Part print with two shaded views. Sizes in mm from the minimum x, y, z corner. Round coordinates to 2 decimals unless told otherwise and drop trailing zeros. Loops run counter-clockwise (first coordinate to the right, second up) from the corner with the lowest first, then second, coordinate; pieces in that order, holes last. Notation, with made-up numbers: (-33.5, 79) -> (22.5, 79) arc R24 ccw to (22.5, 100) -> close; hole circle Ø6 at (32, 41). An arc over 180 degrees is marked (long way). Use a Markdown table: item, result. Add a question column.
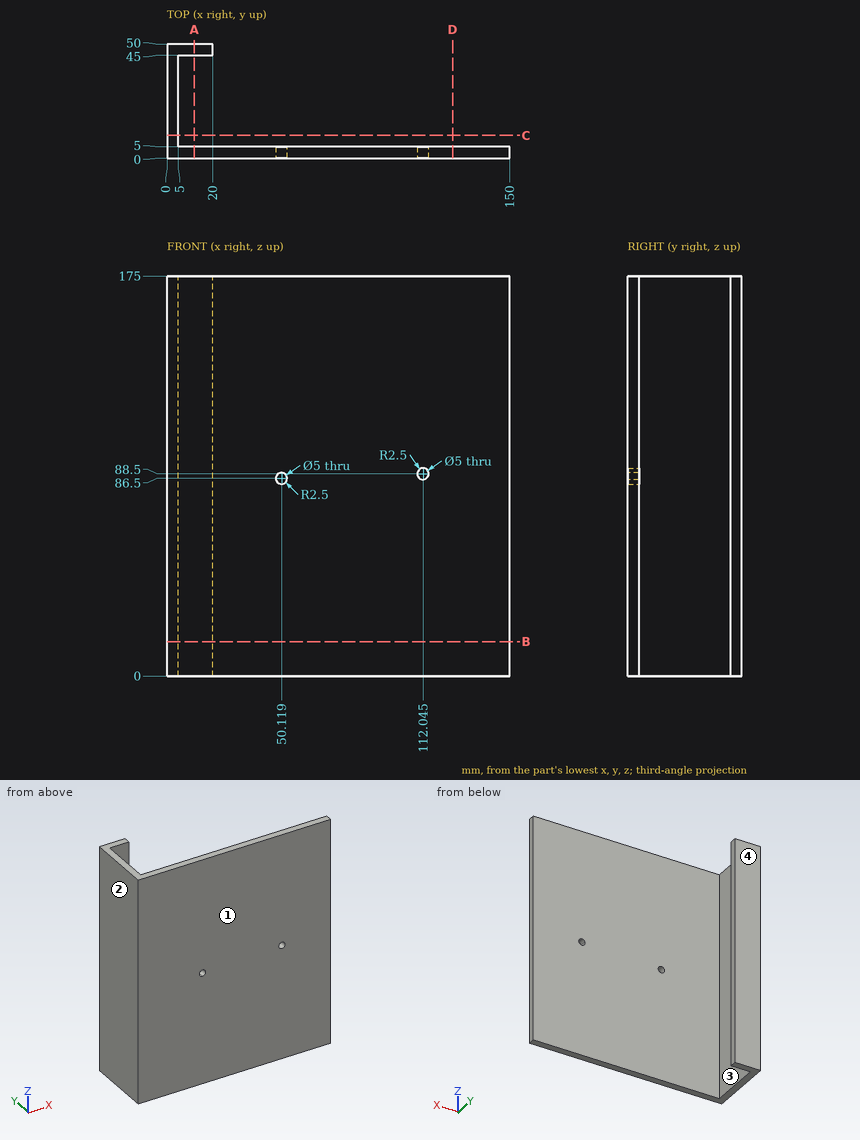
1) Cut at A-A on x = 12. Write the cut outline in (y, z).
2) Pull direction Y, two halves, no side cores. Call the marked faces 1, 2, 3 and 4: +Y half, -Y half, draft (parallel to the pull), parting line (faces both ways), or undercut.
3) Cut at B-B on z = 15. Write the cut outline in (x, y), and give its area (3 significant figures).
4) Cut at C-C on y = 10. Write the cut outline in (x, z), and give its area (3 significant figures).
5) Wall check: probe 1 along X at (y, z) = (2, 88.5) (1 decimal); probe 2 along X at (y, z) = (2, 88) (1 decimal); probe 3 along Y at (x, z) = (130.5, 32). Give the ranges that are in metal, low to high. Write a range as from..to.
6) Pin check, flat tips, straight feed: pin 1 Ø12 at (y, z) = (27.5, 135) entering from -X; pin 2 Ø20 at (y, z) = (19.5, 56) entering from +X; pin 3 Ø4 at (y, z) = (48, 61) entering from +X; pin 4 Ø8 at (x, z) = (57.5, 151.5) entering from +Y. Stop position of each tip, or through.
Established:
| question | item | result |
|---|---|---|
| 1 | outline | (0, 0) -> (5, 0) -> (5, 175) -> (0, 175) -> close; (45, 0) -> (50, 0) -> (50, 175) -> (45, 175) -> close |
| 2 | face 1 | -Y half |
| 2 | face 2 | draft |
| 2 | face 3 | undercut |
| 2 | face 4 | +Y half |
| 3 | outline | (0, 0) -> (150, 0) -> (150, 5) -> (5, 5) -> (5, 45) -> (20, 45) -> (20, 50) -> (0, 50) -> close |
| 3 | area | 1,050 mm^2 |
| 4 | outline | (0, 0) -> (5, 0) -> (5, 175) -> (0, 175) -> close |
| 4 | area | 875 mm^2 |
| 5 | probe 1 | x = 0..48.6, 51.6..109.5, 114.5..150 |
| 5 | probe 2 | x = 0..48.1, 52.1..109.6, 114.5..150 |
| 5 | probe 3 | y = 0..5 |
| 6 | pin 1 | stops at x = 0 |
| 6 | pin 2 | stops at x = 5 |
| 6 | pin 3 | stops at x = 20 |
| 6 | pin 4 | stops at y = 5 |
